Autodesk Inventor part; units mm, degrees
ref_plane "YZ Plane" through (0, 0, 0) normal (1, 0, 0) x (0, 1, 0)
ref_plane "XZ Plane" through (0, 0, 0) normal (0, 1, 0) x (-1, 0, 0)
ref_plane "XY Plane" through (0, 0, 0) normal (0, 0, 1) x (1, 0, 0)
sketch "Sketch1" plane through (0, 0, 0) normal (0, 1, 0) x (-1, 0, 0)
  line L0 (0, 7.3323) -> (6.35, 3.6662)
  line L1 (6.35, 3.6662) -> (6.35, -3.6662)
  line L2 (6.35, -3.6662) -> (0, -7.3323)
  line L3 (0, -7.3323) -> (-6.35, -3.6662)
  line L4 (-6.35, -3.6662) -> (-6.35, 3.6662)
  line L5 (-6.35, 3.6662) -> (0, 7.3323)
  point P0 (0, 0)
  point P1 (0, 0)
  dimension "d0" = 12.7
extrude "Extrusion1" add sketch "Sketch1" along normal blind 32
sketch "Sketch2" plane through (0, 0, 0) normal (0, -1, 0) x (1, 0, 0)
  circle A0 centre (0, 0) radius 4
  dimension "d3" = 8
extrude "Extrusion2" add sketch "Sketch2" along normal blind 30
sketch "Sketch3" plane through (0, -30, 0) normal (0, -1, 0) x (1, 0, 0)
  point P0 (0, 0)
hole "Hole1" at (0, -30, 0) direction (0, 1, 0) diameter 4.917 depth 17.1 tip angle 118
properties part number "Axle"
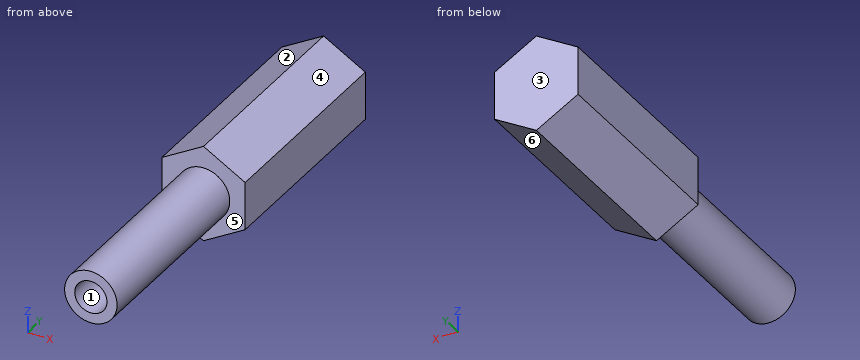
The listing builds one solid part. Answer for the finished solid, in the listing's coordinates (mm). Face numbers are marked on the shaded views. A direction names the side the tool comes from. Coordinates: 2 decimals unless noted, no trailing zeros. Loops run counter-clockwise (first coordinate to the right, second up) from the corner with the lowest first, then second, coordinate; pieces in that order, holes last.
1) Determine the mould class of the marked faces 1, 2, 3 and 4 for opening direction X: pulls with the +X half, pulls with the -X half, needs draft (parallel to the pull), parting line crosses it, or undercut.
2) Find section A-A on y = 6. Write down the section's boundary in (x, z), then the cut area to 3 significant figures.
3) Find section D-D on y = -9.5. Write down the section's boundary in (x, z).
4) Flat-ended cylindrical pins translate along their axes: pin 1 Ø4 at (x, z) = (0, 0) entering from -Y; pin 2 Ø1 at (y, z) = (-2.5, 4) entering from +X; pin 3 Ø8 at (y, z) = (-21.5, 3.5) entering from -X. Find the tip coordinate at first contact, or state that the pin passes through.
5) A tool of negligible diameter and unlimited length cuts with its end or side. For the marked faces 5 and 6, from which of +Z, -Z, +X, -X, +Y, -Y can it reach the whole face along a straight path? Write none if from no direction.
6) Find section B-B on x = 5.75. Write down the section's boundary in (y, z).
7) Find section C-C on z = -5.5. Write down the section's boundary in (x, y), then the cut area to 3 significant figures.
8) Find the intervals of material crossed by L1, parallel to Z at x = 0, y = -20; L2, parallel to Y at x = 3.5, z = 4.25, in increasing order.
Values:
1. face 1: undercut
1. face 2: pulls with the -X half
1. face 3: needs draft
1. face 4: pulls with the +X half
2. outline: (-6.35, -3.67) - (0, -7.33) - (6.35, -3.67) - (6.35, 3.67) - (0, 7.33) - (-6.35, 3.67) - close
2. area: 140 mm2
3. outline: circle Ø8 at (0, 0)
4. pin 1: stops at y = -12.62
4. pin 2: stops at x = 1.94
4. pin 3: stops at x = -4
5. face 5: -Y
5. face 6: -Z, +X, +Y, -Y
6. outline: (0, -4.01) - (32, -4.01) - (32, 4.01) - (0, 4.01) - close
7. outline: (-3.17, 0) - (3.17, 0) - (3.17, 32) - (-3.17, 32) - close
7. area: 203 mm2
8. L1: z = -4 to -2.46, 2.46 to 4
8. L2: y = 0 to 32
